from build123d import *

# Parameters (mm, degrees)
CROQUIS1_R                 = 55
SALIENTE_EXTRUIR1_DEPTH    = 92
CROQUIS2_W                 = 287.965144552
CROQUIS2_H                 = 82
SALIENTE_EXTRUIR2_DEPTH    = 92
CROQUIS5_W                 = 372
CROQUIS5_H                 = 8
SALIENTE_EXTRUIR5_DEPTH    = 10
SALIENTE_EXTRUIR6_START    = -77
SALIENTE_EXTRUIR6_DEPTH    = 77
VACIADO1_START             = -28.5
VACIADO1_DEPTH             = 57
VACIADO1_START_2           = 10
VACIADO1_2_DEPTH           = 72
CROQUIS8_W                 = 26
CROQUIS8_H                 = 190
SALIENTE_EXTRUIR7_DEPTH    = 10
CROQUIS9_W                 = 26
CROQUIS9_H                 = 190
SALIENTE_EXTRUIR8_DEPTH    = 10
SALIENTE_EXTRUIR9_DEPTH    = 61
CORTAR_EXTRUIR1_DEPTH      = 69
CORTAR_EXTRUIR1_DEPTH_BACK = 16
CORTAR_EXTRUIR2_DEPTH      = 514.698364466
CORTAR_EXTRUIR2_DEPTH_BACK = 514.698364466
CROQUIS14_R                = 4.5
VACIADO4_START             = -354.625750112
VACIADO4_OUTLINE_W         = 41
VACIADO4_OUTLINE_H         = 238
VACIADO4_DEPTH             = 20
CROQUIS15_W                = 45
CROQUIS15_H                = 41
SALIENTE_EXTRUIR10_DEPTH   = 30


# Read off the part's stored shape, not the designer's step: Vaciado1, Vaciado4
with BuildPart() as part:
    # Croquis1 → Saliente-Extruir1 (new body)
    with BuildSketch(Plane.XY):
        Circle(CROQUIS1_R)
    extrude(amount=SALIENTE_EXTRUIR1_DEPTH)

    # Croquis2 → Saliente-Extruir2 (add)
    with BuildSketch(Plane(origin=(0, 0, 0), x_dir=(-1, 0, 0), z_dir=(0, 0, -1))):
        with Locations((180.643177836, 0)):
            Rectangle(CROQUIS2_W, CROQUIS2_H)
    extrude(amount=-SALIENTE_EXTRUIR2_DEPTH)

    # Croquis5 → Saliente-Extruir5 (add)
    with BuildSketch(Plane.ZY.offset(324.625750112)):
        with Locations((212, 34.5)):
            Rectangle(CROQUIS5_W, CROQUIS5_H)
        with Locations((212, -34.5)):
            Rectangle(CROQUIS5_W, CROQUIS5_H)
    extrude(amount=SALIENTE_EXTRUIR5_DEPTH)

    # Croquis6 → Saliente-Extruir6 (add)
    with BuildSketch(Plane.XZ.offset(38.5).offset(SALIENTE_EXTRUIR6_START)):
        Polygon((-324.625750112, 216), (-224.625750112, 216), (-187.625750112, 227.033203383), (-187.625750112, 339), (-254.625750112, 339), (-254.625750112, 403), (-324.625750112, 403), align=None)
    extrude(amount=SALIENTE_EXTRUIR6_DEPTH)

    # Vaciado1 outline → Vaciado1 (cut)
    with BuildSketch(Plane(origin=(0, 0, 0), x_dir=(1, 0, 0), z_dir=(0, 1, 0)).offset(VACIADO1_START)):
        Polygon((-197.625750112, -234.486389827), (-226.08497566, -226), (-324.625750112, -226), (-324.625750112, -393), (-264.625750112, -393), (-264.625750112, -329), (-197.625750112, -329), align=None)
    extrude(amount=VACIADO1_DEPTH, mode=Mode.SUBTRACT)

    # Vaciado1 2 outline → Vaciado1 2 (cut)
    with BuildSketch(Plane.XY.offset(VACIADO1_START_2)):
        with BuildLine():
            Line((-32.619012861, 31), (-314.625750112, 31))
            Line((-314.625750112, 31), (-314.625750112, -31))
            Line((-314.625750112, -31), (-32.619012861, -31))
            ThreePointArc((-32.619012861, -31), (45, 0), (-32.619012861, 31))
        make_face()
    extrude(amount=VACIADO1_2_DEPTH, mode=Mode.SUBTRACT)

    # Croquis8 → Saliente-Extruir7 (add)
    with BuildSketch(Plane(origin=(0, 38.5, 0), x_dir=(1, 0, 0), z_dir=(0, 1, 0))):
        with Locations((-321.625750112, -316)):
            Rectangle(CROQUIS8_W, CROQUIS8_H)
    extrude(amount=SALIENTE_EXTRUIR7_DEPTH)

    # Croquis9 → Saliente-Extruir8 (add)
    with BuildSketch(Plane.XZ.offset(38.5)):
        with Locations((-321.625750112, 316)):
            Rectangle(CROQUIS9_W, CROQUIS9_H)
    extrude(amount=SALIENTE_EXTRUIR8_DEPTH)

    # Croquis10 → Saliente-Extruir9 (add)
    with BuildSketch(Plane.XZ.offset(-30.5)):
        Polygon((-324.625750112, 86), (-377.625750112, 86), (-377.625750112, 104), (-354.625750112, 104), (-354.625750112, 334), (-324.625750112, 334), align=None)
    extrude(amount=SALIENTE_EXTRUIR9_DEPTH)

    # Croquis11 → Revolución1 (revolve)
    with BuildSketch(Plane.ZY.offset(377.625750112)):
        Polygon((110, 0), (110, 30), (42, 30), (34, 35), (22, 35), (22, 0), align=None)
    revolve(axis=Axis((-377.625750112, 0, 0), (0, 0, 1)))

    # Croquis13 → Cortar-Extruir1 (cut, two sides: drawn at the far end of the back side and taken through both)
    with BuildSketch(Plane.ZY.offset(354.625750112).offset(-CORTAR_EXTRUIR1_DEPTH_BACK)):
        Polygon((48.064346335, 30.5), (14.405684341, 30.5), (14.405684341, 38.395591982), (46.194420669, 38.5), align=None)
        Polygon((43.319665348, -30.5), (18.175664467, -30.5), (19.260307642, -37.859564216), (38.945879671, -34.958329751), align=None)
    extrude(amount=CORTAR_EXTRUIR1_DEPTH + CORTAR_EXTRUIR1_DEPTH_BACK, mode=Mode.SUBTRACT)

    # Croquis14 → Cortar-Extruir2 (cut, two sides: drawn at the far end of the back side and taken through both)
    with BuildSketch(Plane.XY.offset(110).offset(-CORTAR_EXTRUIR2_DEPTH_BACK)):
        with Locations(Location((-377.625750112, 0, 0), (0, 0, 90))):
            Circle(CROQUIS14_R)
    extrude(amount=CORTAR_EXTRUIR2_DEPTH + CORTAR_EXTRUIR2_DEPTH_BACK, mode=Mode.SUBTRACT)

    # Vaciado4 outline → Vaciado4 (cut)
    with BuildSketch(Plane.YZ.offset(VACIADO4_START)):
        with Locations((0, 215)):
            Rectangle(VACIADO4_OUTLINE_W, VACIADO4_OUTLINE_H)
    extrude(amount=VACIADO4_DEPTH, mode=Mode.SUBTRACT)

    # Croquis15 → Saliente-Extruir10 (add)
    with BuildSketch(Plane.ZY.offset(324.625750112)):
        with Locations((48.5, 0)):
            Rectangle(CROQUIS15_W, CROQUIS15_H)
    extrude(amount=SALIENTE_EXTRUIR10_DEPTH)


solid = part.part
Input: part model. Units: mm. Frame: model coordinates. A direction names the side the tool comes from. Coordinates: 2 decimals unless noted, no trailing zeros. Loops run counter-clockwise (first coordinate to the right, second up) from the corner with the lowest first, then second, coordinate; pieces in that order, holes last.
Q1. Draft query along Z for faces 6 (the face through (-322, 43, 411)), 7 (the face through (-324.626, 1, 153)), 8 (the face through (-377, -30.5, 30)). Return one class per face: +Z half, -Z half, draft (parallel to the pull), parting line (faces both ways), or undercut.
Q2. Cut plane B-B (z = 271). Output: boundary loops of the cut face in (x, y).
Q3. Contact query for flat-ended pins moving along their axis: pin 1 (5 mm diameter, centred on y = -27, z = 258.5, fed in from -X); pin 2 (11 mm diameter, centred on x = -328, y = 42, fed in from -Z); pin 3 (5 mm diameter, centred on y = -28.5, z = 87, fed in from +X); pin 4 (1 mm diameter, centred on x = -84, z = 73.5, fed in from -Y). Output: stop coordinate, or through.
Q4. Cut plane C-C (z = 348). Output: boundary loops of the cut face in (x, y).
Q5. Cut plane D-D (x = 0). Output: boundary loops of the cut face in (y, z), then the cut area to 3 significant figures.
Q6. Cut plane A-A (x = -54). Output: boundary loops of the cut face in (y, z), then the cut area to 3 significant figures.
Q7. Set-up query: faces 1 (the face through (-322, 43, 221)), 2 (the face through (-334.626, 37, 264)), 3 (the face through (-137, 1, 82)), 4 (the face through (-308.626, 43, 317)), 5 (the face through (-354.626, 0, 103)). Return all of +Z, -Z, +X, -X, +Y, -Y with unobstructed straight access to the full face (end or side cutting, diameter ignored); none if empty.
Q8. Material intervals for line 1 (X direction, y = 0, z = 84.5); line 2 (Z direction, x = -272, y = -17); line 3 (X direction, y = 0, z = 48), sorted ascending.
Working result:
1. face 6: +Z half
1. face 7: undercut
1. face 8: draft
2. outline: (-354.63, -30.5) - (-334.63, -30.5) - (-334.63, -48.5) - (-308.63, -48.5) - (-308.63, -38.5) - (-187.63, -38.5) - (-187.63, 38.5) - (-308.63, 38.5) - (-308.63, 48.5) - (-334.63, 48.5) - (-334.63, 30.5) - (-354.63, 30.5) - (-354.63, 20.5) - (-334.63, 20.5) - (-334.63, -20.5) - (-354.63, -20.5) - close; hole (-324.63, -28.5) - (-197.63, -28.5) - (-197.63, 28.5) - (-324.63, 28.5) - close
3. pin 1: stops at x = -354.63
3. pin 2: stops at z = 0
3. pin 3: stops at x = 48.47
3. pin 4: stops at y = -41
4. outline: (-334.63, -48.5) - (-308.63, -48.5) - (-308.63, -38.5) - (-254.63, -38.5) - (-254.63, 38.5) - (-308.63, 38.5) - (-308.63, 48.5) - (-334.63, 48.5) - (-334.63, 30.5) - (-324.63, 30.5) - (-324.63, 28.5) - (-264.63, 28.5) - (-264.63, -28.5) - (-324.63, -28.5) - (-324.63, -30.5) - (-334.63, -30.5) - close
5. outline: (-55, 0) - (55, 0) - (55, 92) - (-55, 92) - close; hole (-45, 10) - (45, 10) - (45, 82) - (-45, 82) - close
5. area: 3,640 mm2
6. outline: (-41, 0) - (41, 0) - (41, 92) - (-41, 92) - close; hole (-31, 10) - (31, 10) - (31, 82) - (-31, 82) - close
6. area: 3,080 mm2
7. face 1: +X, -X, +Y
7. face 2: +Z, -Z, -X, +Y
7. face 3: none
7. face 4: +Z, +X, +Y
7. face 5: +Z
8. line 1: x = -407.63 to -382.13, -373.13 to -347.63, -324.63 to 55
8. line 2: z = 0 to 10, 82 to 92, 216 to 226, 393 to 403
8. line 3: x = -407.63 to -382.13, -373.13 to -314.63, 45 to 55
